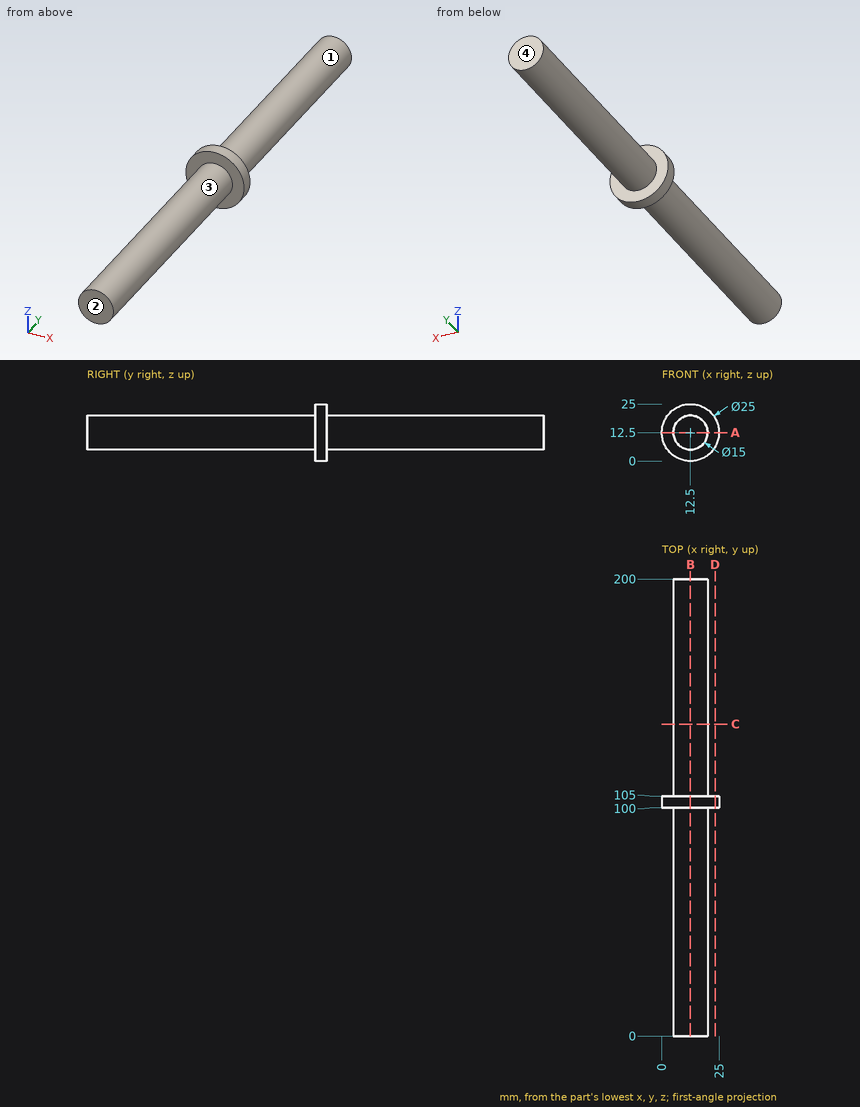
Could you check a few things on this drawing? It's one solid part, dimensions in mm from its lowest x, y, z. A direction names the side the tool comes from. Coordinates: 2 decimals unless noted, no trailing zeros. Order: outer loops, then holes, each group sorted by start corner. A loop starts at its lowest first (then second) coordinate and runs counter-clockwise, first axis right, second up. Notation, with made-up numbers: (44, -15.75) - (54, -15.75) arc R22 ccw to (54, -6.75) - close; hole circle Ø10 at (84, 23). An arc over 180 degrees is marked (long way). Answer as a JSON object with one key per item and string values. Group by question number.
Q1. Will these pins go through, and if not, where does the flat tip stop? P1, Ø10, axis at y = 110.5, z = 5.5, coming from the -X side; P2, Ø4, axis at y = 59, z = 7.5, coming from the -X side; P3, Ø12, axis at x = 10, y = 149, coming from the +Z side.
Q2. On a 3-axis mill with a long thin cutter (end or side, diameter ignored), from which of +Z, -Z, +X, -X, +Y, -Y can I reach the whole of each face in a straight line? I mean the marked faces 3 and 4. Say none if no direction works.
Q3. Imagine slicing it at C-C (y = 136.5). Please give me the cut outline in (x, z).
Q4. Imagine slicing it at A-A (z = 12.5). Please give me the cut outline in (x, y).
Q5. I need wall thicknesses on line 1 (Y direction, x = 16.25, z = 4); line 2 (Z direction, x = 10.5, y = 102.5); line 3 (X direction, y = 151, z = 9). Which ranges of each line are inside material? Lowest first, please. Write a range as from..to.
Q6. Imagine slicing it at B-B (x = 12.5). Please give me the cut outline in (y, z).
Q7. We'd pull the mould along Z, two halves only. Please class the marked faces 1 and 2: +Z half, -Z half, draft (parallel to the pull), parting line (faces both ways), or undercut.
Q8. Imagine slicing it at D-D (x = 23.25). Please give me the cut outline in (y, z).
Determined:
{
 "1": {"P1": "stops at x = 5.27", "P2": "stops at x = 5.63", "P3": "stops at z = 20"},
 "2": {"face 3": "-Y", "face 4": "+Z, -Z, +X, -X, +Y"},
 "3": {"outline": "circle Ø15 at (12.5, 12.5)"},
 "4": {"outline": "(0, 100) - (5, 100) - (5, 0) - (20, 0) - (20, 100) - (25, 100) - (25, 105) - (20, 105) - (20, 200) - (5, 200) - (5, 105) - (0, 105) - close"},
 "5": {"line 1": "y = 100..105", "line 2": "z = 0.16..24.84", "line 3": "x = 5.87..19.13"},
 "6": {"outline": "(0, 5) - (100, 5) - (100, 0) - (105, 0) - (105, 5) - (200, 5) - (200, 20) - (105, 20) - (105, 25) - (100, 25) - (100, 20) - (0, 20) - close"},
 "7": {"face 1": "parting line", "face 2": "draft"},
 "8": {"outline": "(100, 6.12) - (105, 6.12) - (105, 18.88) - (100, 18.88) - close"}
}
